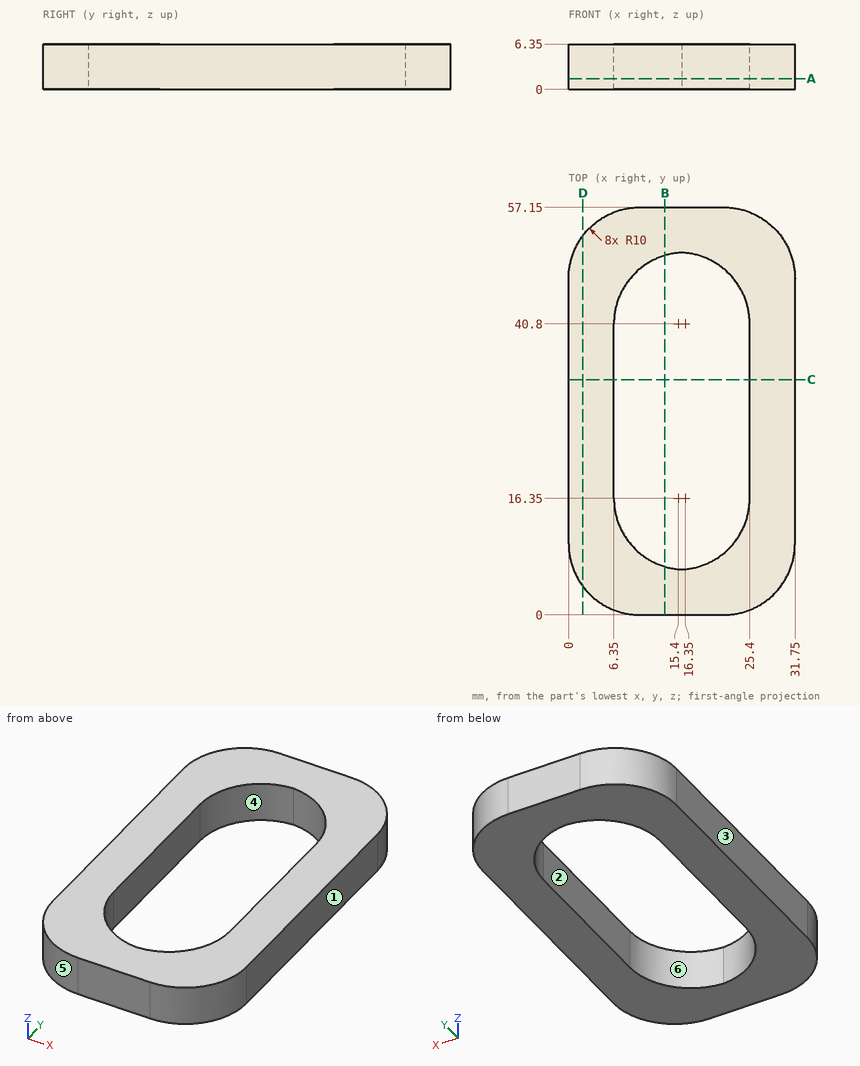
Drawing for the job (mm, zero at the part's lowest x, y, z). A direction names the side the tool comes from. Round coordinates to 2 decimals unless told otherwise and drop trailing zeros. Write each loop counter-clockwise with the first axis right and the second up, starting at its lowest first coordinate (ties: lowest second). Pieces come first, ordered by that corner, then holes.
Item 1: Drill centre lines: L1, parallel to X at y = 32, z = 5.25; L2, parallel to Y at x = 19.5, z = 4; L3, parallel to Y at x = 15.5, z = 1.25. Where is each one in solid material? Low to high.
Filled in:
L1: x = 0 to 6.35, 25.4 to 31.75
L2: y = 0 to 7.23, 49.92 to 57.15
L3: y = 0 to 6.39, 50.76 to 57.15
Item 2: Drop a flat-ended pin along its axis: pin 1 Ø3 at (y, z) = (50, 4.5) entering from +X. Give the stop position or say it passes through.
Filled in:
pin 1: stops at x = 31.66
Item 3: Tool access for the marked faces 5 and 6: list every direction of +Z, -Z, +X, -X, +Y, -Y with a clear straight run to the whole face (end or side of a thin tool).
Filled in:
face 5: +Z, -Z, -X, -Y
face 6: +Z, -Z
Item 4: Band-saw the part on B-B on x = 13.5. Write the cut outline in (y, z).
Filled in:
outline: (0, 0) - (6.76, 0) - (6.76, 6.35) - (0, 6.35) - close; (50.39, 0) - (57.15, 0) - (57.15, 6.35) - (50.39, 6.35) - close
Item 5: Band-saw the part on A-A on z = 1.5. Write the cut outline in (x, y) (3 decimals).
Filled in:
outline: (0, 10) arc R10 ccw to (10, 0) - (21.75, 0) arc R10 ccw to (31.75, 10) - (31.75, 47.15) arc R10 ccw to (21.75, 57.15) - (10, 57.15) arc R10 ccw to (0, 47.15) - close; hole (6.35, 16.35) arc R10 ccw to (15.875, 6.361) arc R10 ccw to (25.4, 16.35) - (25.4, 40.8) arc R10 ccw to (15.875, 50.789) arc R10 ccw to (6.35, 40.8) - close
Item 6: Mould opens along X. For the marked faces 1, 2, 3 and 4 say: released by +X, released by -X, zero draft, split by the parting line, or undercut.
Filled in:
face 1: released by +X
face 2: undercut
face 3: released by -X
face 4: undercut
Item 7: Band-saw the part on C-C on y = 33. Write the cut outline in (x, z).
Filled in:
outline: (0, 0) - (6.35, 0) - (6.35, 6.35) - (0, 6.35) - close; (25.4, 0) - (31.75, 0) - (31.75, 6.35) - (25.4, 6.35) - close
Item 8: Band-saw the part on D-D on x = 2. Write the cut outline in (y, z), then the cut area to 3 significant figures.
Filled in:
outline: (4, 0) - (53.15, 0) - (53.15, 6.35) - (4, 6.35) - close
area: 312 mm2
